from build123d import *

# Parameters (mm, degrees)
BOSS_EXTRUDE1_DEPTH  = 80
BOSS_EXTRUDE2_DEPTH  = 6
BOSS_EXTRUDE3_DEPTH  = 6
CUT_EXTRUDE1_REACH   = 93.829
SKETCH6_W            = 14
SKETCH6_H            = 10
CUT_EXTRUDE2_DEPTH   = 6
BOSS_EXTRUDE4_DEPTH  = 10
BOSS_EXTRUDE11_DEPTH = 10
CUT_EXTRUDE3_REACH   = 113.919
SKETCH9_R            = 1.5


with BuildPart() as part:
    # Sketch1 → Boss-Extrude1 (new body)
    with BuildSketch(Plane(origin=(0, 0, 0), x_dir=(0, 0, -1), z_dir=(1, 0, 0))):
        Polygon((0, 0), (40, 0), (40, 12), (38.5, 12), (38.5, 6), (25, 6), (25, 12), (23.5, 12), (23.5, 6), (16.5, 6), (16.5, 12), (15, 12), (15, 6), (1.5, 6), (1.5, 12), (0, 12), align=None)
    extrude(amount=BOSS_EXTRUDE1_DEPTH)

    # Sketch2 → Boss-Extrude2 (add)
    with BuildSketch(Plane(origin=(6.2, 0, 0), x_dir=(0, 0, -1), z_dir=(1, 0, 0))):
        Polygon((15, 6), (15, 12), (9, 15), (9, 20.8), (31, 20.8), (31, 15), (25, 12), (25, 6), align=None)
    extrude(amount=-BOSS_EXTRUDE2_DEPTH)

    # Sketch4 → Boss-Extrude3 (add)
    with BuildSketch(Plane(origin=(47, 0, 0), x_dir=(0, 0, -1), z_dir=(1, 0, 0))):
        Polygon((25, 6), (15, 6), (15, 12), (9, 15), (9, 20.8), (31, 20.8), (31, 15), (25, 12), align=None)
    extrude(amount=BOSS_EXTRUDE3_DEPTH)

    # Sketch5 → Cut-Extrude1 (cut, up to next)
    with BuildSketch(Plane.XZ, mode=Mode.PRIVATE) as cut_extrude1_sk1:
        with BuildLine():
            Line((8, -31), (72, -31))
            ThreePointArc((72, -31), (74.5, -33.5), (72, -36))
            Line((72, -36), (8, -36))
            ThreePointArc((8, -36), (5.5, -33.5), (8, -31))
        make_face()
    cut_extrude1_tool1 = extrude(cut_extrude1_sk1.sketch, amount=-CUT_EXTRUDE1_REACH, mode=Mode.PRIVATE) & part.part
    # Sketch5 → Cut-Extrude1 (cut, up to next)
    with BuildSketch(Plane.XZ, mode=Mode.PRIVATE) as cut_extrude1_sk2:
        with BuildLine():
            Line((72, -4), (8, -4))
            ThreePointArc((8, -4), (5.5, -6.5), (8, -9))
            Line((8, -9), (72, -9))
            ThreePointArc((72, -9), (74.5, -6.5), (72, -4))
        make_face()
    cut_extrude1_tool2 = extrude(cut_extrude1_sk2.sketch, amount=-CUT_EXTRUDE1_REACH, mode=Mode.PRIVATE) & part.part
    add(cut_extrude1_tool1.solids().sort_by_distance((40, 0, -33.5))[0], mode=Mode.SUBTRACT)
    add(cut_extrude1_tool2.solids().sort_by_distance((40, 0, -6.5))[0], mode=Mode.SUBTRACT)

    # Sketch6 → Cut-Extrude2 (cut)
    with BuildSketch(Plane(origin=(0, 6, 0), x_dir=(1, 0, 0), z_dir=(0, 1, 0))):
        with Locations((40, 20)):
            Rectangle(SKETCH6_W, SKETCH6_H)
    extrude(amount=CUT_EXTRUDE2_DEPTH, mode=Mode.SUBTRACT)

    # Sketch7 → Boss-Extrude4 (add)
    with BuildSketch(Plane(origin=(80, 0, 0), x_dir=(0, 0, -1), z_dir=(1, 0, 0))):
        Polygon((0, 0), (40, 0), (40, 12), (40, 53.158651342), (10, 53.158651342), (0, 12), align=None)
        Polygon((35, 48.158651342), (13.930649368, 48.158651342), (8.463997944, 25.658651342), (35, 25.658651342), align=None, mode=Mode.SUBTRACT)
        Polygon((35, 20.8), (7.283528909, 20.8), (5.145460796, 12), (35, 12), align=None, mode=Mode.SUBTRACT)
    extrude(amount=BOSS_EXTRUDE4_DEPTH)

    # Sketch8 → Boss-Extrude11 (add)
    with BuildSketch(Plane.ZY):
        Polygon((0, 12), (0, 0), (-40, 0), (-40, 12), (-40, 53.158651342), (-10, 53.158651342), align=None)
        Polygon((-5.145460796, 12), (-35, 12), (-35, 20.8), (-7.283528909, 20.8), align=None, mode=Mode.SUBTRACT)
        Polygon((-13.930649368, 48.158651342), (-8.463997944, 25.658651342), (-35, 25.658651342), (-35, 48.158651342), align=None, mode=Mode.SUBTRACT)
    extrude(amount=BOSS_EXTRUDE11_DEPTH)

    # Sketch9 → Cut-Extrude3 (cut, up to next)
    with BuildSketch(Plane(origin=(0, 0, -40), x_dir=(-1, 0, 0), z_dir=(0, 0, -1)), mode=Mode.PRIVATE) as cut_extrude3_sk1:
        with Locations((-85, 43.158651342)):
            Circle(SKETCH9_R)
    cut_extrude3_tool1 = extrude(cut_extrude3_sk1.sketch, amount=-CUT_EXTRUDE3_REACH, mode=Mode.PRIVATE) & part.part
    # Sketch9 → Cut-Extrude3 (cut, up to next)
    with BuildSketch(Plane(origin=(0, 0, -40), x_dir=(-1, 0, 0), z_dir=(0, 0, -1)), mode=Mode.PRIVATE) as cut_extrude3_sk2:
        with Locations((-85, 30.658651342)):
            Circle(SKETCH9_R)
    cut_extrude3_tool2 = extrude(cut_extrude3_sk2.sketch, amount=-CUT_EXTRUDE3_REACH, mode=Mode.PRIVATE) & part.part
    # Sketch9 → Cut-Extrude3 (cut, up to next)
    with BuildSketch(Plane(origin=(0, 0, -40), x_dir=(-1, 0, 0), z_dir=(0, 0, -1)), mode=Mode.PRIVATE) as cut_extrude3_sk3:
        with Locations((-85, 15.658651342)):
            Circle(SKETCH9_R)
    cut_extrude3_tool3 = extrude(cut_extrude3_sk3.sketch, amount=-CUT_EXTRUDE3_REACH, mode=Mode.PRIVATE) & part.part
    # Sketch9 → Cut-Extrude3 (cut, up to next)
    with BuildSketch(Plane(origin=(0, 0, -40), x_dir=(-1, 0, 0), z_dir=(0, 0, -1)), mode=Mode.PRIVATE) as cut_extrude3_sk4:
        with Locations((5, 43.158651342)):
            Circle(SKETCH9_R)
    cut_extrude3_tool4 = extrude(cut_extrude3_sk4.sketch, amount=-CUT_EXTRUDE3_REACH, mode=Mode.PRIVATE) & part.part
    # Sketch9 → Cut-Extrude3 (cut, up to next)
    with BuildSketch(Plane(origin=(0, 0, -40), x_dir=(-1, 0, 0), z_dir=(0, 0, -1)), mode=Mode.PRIVATE) as cut_extrude3_sk5:
        with Locations((5, 30.658651342)):
            Circle(SKETCH9_R)
    cut_extrude3_tool5 = extrude(cut_extrude3_sk5.sketch, amount=-CUT_EXTRUDE3_REACH, mode=Mode.PRIVATE) & part.part
    # Sketch9 → Cut-Extrude3 (cut, up to next)
    with BuildSketch(Plane(origin=(0, 0, -40), x_dir=(-1, 0, 0), z_dir=(0, 0, -1)), mode=Mode.PRIVATE) as cut_extrude3_sk6:
        with Locations((5, 15.658651342)):
            Circle(SKETCH9_R)
    cut_extrude3_tool6 = extrude(cut_extrude3_sk6.sketch, amount=-CUT_EXTRUDE3_REACH, mode=Mode.PRIVATE) & part.part
    add(cut_extrude3_tool1.solids().sort_by_distance((85, 43.158651, -40))[0], mode=Mode.SUBTRACT)
    add(cut_extrude3_tool2.solids().sort_by_distance((85, 30.658651, -40))[0], mode=Mode.SUBTRACT)
    add(cut_extrude3_tool3.solids().sort_by_distance((85, 15.658651, -40))[0], mode=Mode.SUBTRACT)
    add(cut_extrude3_tool4.solids().sort_by_distance((-5, 43.158651, -40))[0], mode=Mode.SUBTRACT)
    add(cut_extrude3_tool5.solids().sort_by_distance((-5, 30.658651, -40))[0], mode=Mode.SUBTRACT)
    add(cut_extrude3_tool6.solids().sort_by_distance((-5, 15.658651, -40))[0], mode=Mode.SUBTRACT)


solid = part.part
Work out the finished part from the listing and answer in its coordinate system (mm). A direction names the side the tool comes from. Give positions to 0.01 mm unless a question says otherwise; leave off trailing zeros. Loops run counter-clockwise (first coordinate to the right, second up) from the corner with the lowest first, then second, coordinate; pieces in that order, holes last. Notation, with made-up numbers: (-31, -10) -> (-6, -10) arc R24 ccw to (-6, 7) -> close; hole circle Ø5 at (-26, -28.5). An arc over 180 degrees is marked (long way). Use a Markdown table: item, result. Add a question column.
1. Determine the mould class of faces 1 (the flat face through (50, 18, -9)), 2 (the flat face through (19, 9, -16.5)), 3 (the cylindrical face through (-4.805, 44.646, -37.535)) for opening direction Z: released by +Z, released by -Z, zero draft, split by the parting line, or undercut.
2. Section D-D on y = 9 is taken. Determine the outline of the cut face in (x, z), and give its area (3 significant figures).
3. Section C-C on x = 26 is taken. Determine the outline of the cut face in (y, z).
4. Flat-ended cylindrical pins translate along their axes: pin 1 Ø4.5 at (x, y) = (4.5, 17.5) entering from -Z; pin 2 Ø2 at (y, z) = (14, -33.5) entering from +X; pin 3 Ø0.8 at (x, z) = (47.5, -39) entering from +Y; pin 4 Ø11 at (x, y) = (85, 31.5) entering from +Z. Find the tip coordinate at first contact, or state that the pin passes through.
5. Section B-B on x = -5 is taken. Determine the outline of the cut face in (y, z), and give its area (3 significant figures).
6. Section A-A on z = -33.5 is taken. Determine the outline of the cut face in (x, y).
7. Find the intervals of material crossed by probe 1 along Z at (x, y) = (73, 11.5); probe 2 along Y at (x, z) = (85, -38.9); probe 3 along Z at (x, y) = (61.5, 5), in increasing order.
8. For faces 4 (the flat face through (17, 9, -15)), 5 (the flat face through (40, 3, -31)), 6 (the flat face through (50, 20.8, -20)), 7 (the flat face through (0, 9, -20)), 8 (the flat face through (84.93, 37.066, -11.236)), determine the directions among +Z, -Z, +X, -X, +Y, -Y from which every point of the face is accessible in a straight line to the end or side of a thin tool.
Results below:
| question | item | result |
|---|---|---|
| 1 | face 1 | released by +Z |
| 1 | face 2 | undercut |
| 1 | face 3 | zero draft |
| 2 | outline | (-10, -40) -> (90, -40) -> (90, 0) -> (-10, 0) -> close; hole (0, -38.5) -> (80, -38.5) -> (80, -25) -> (47, -25) -> (47, -15) -> (80, -15) -> (80, -1.5) -> (0, -1.5) -> (0, -15) -> (33, -15) -> (33, -16.5) -> (6.2, -16.5) -> (6.2, -23.5) -> (33, -23.5) -> (33, -25) -> (0, -25) -> close; hole (0, -23.5) -> (0.2, -23.5) -> (0.2, -16.5) -> (0, -16.5) -> close; hole (53, -23.5) -> (80, -23.5) -> (80, -16.5) -> (53, -16.5) -> close |
| 2 | area | 1,320 mm^2 |
| 3 | outline | (0, -40) -> (12, -40) -> (12, -38.5) -> (6, -38.5) -> (6, -36) -> (0, -36) -> close; (0, -31) -> (6, -31) -> (6, -25) -> (12, -25) -> (12, -23.5) -> (6, -23.5) -> (6, -16.5) -> (12, -16.5) -> (12, -15) -> (6, -15) -> (6, -9) -> (0, -9) -> close; (0, -4) -> (6, -4) -> (6, -1.5) -> (12, -1.5) -> (12, 0) -> (0, 0) -> close |
| 4 | pin 1 | stops at z = -31 |
| 4 | pin 2 | passes through |
| 4 | pin 3 | stops at y = 12 |
| 4 | pin 4 | stops at z = -3.4 |
| 5 | outline | (0, -40) -> (14.16, -40) -> (14.16, -35) -> (12, -35) -> (12, -5.15) -> (20.8, -7.28) -> (20.8, -35) -> (17.16, -35) -> (17.16, -40) -> (29.16, -40) -> (29.16, -35) -> (25.66, -35) -> (25.66, -8.46) -> (48.16, -13.93) -> (48.16, -35) -> (44.66, -35) -> (44.66, -40) -> (53.16, -40) -> (53.16, -10) -> (12, 0) -> (0, 0) -> close; (32.16, -40) -> (41.66, -40) -> (41.66, -35) -> (32.16, -35) -> close |
| 5 | area | 1,090 mm^2 |
| 6 | outline | (-10, 0) -> (5.5, 0) -> (5.5, 6) -> (0, 6) -> (0, 12) -> (-10, 12) -> close; (-10, 20.8) -> (0, 20.8) -> (0, 25.66) -> (-10, 25.66) -> close; (-10, 48.16) -> (0, 48.16) -> (0, 53.16) -> (-10, 53.16) -> close; (74.5, 0) -> (90, 0) -> (90, 12) -> (80, 12) -> (80, 6) -> (74.5, 6) -> close; (80, 20.8) -> (90, 20.8) -> (90, 25.66) -> (80, 25.66) -> close; (80, 48.16) -> (90, 48.16) -> (90, 53.16) -> (80, 53.16) -> close |
| 7 | probe 1 | z = -40 to -38.5, -25 to -23.5, -16.5 to -15, -1.5 to 0 |
| 7 | probe 2 | y = 0 to 14.16, 17.16 to 29.16, 32.16 to 41.66, 44.66 to 53.16 |
| 7 | probe 3 | z = -40 to -36, -31 to -9, -4 to 0 |
| 8 | face 4 | none |
| 8 | face 5 | +Y, -Y |
| 8 | face 6 | +Z, -Z, +Y |
| 8 | face 7 | +Y |
| 8 | face 8 | +X, -X |
